For this review, use the dimensioned drawing (mm, ordinates from the lowest corner) and the shaded views. Coordinates: 2 decimals unless noted, no trailing zeros. Order: outer loops, then holes, each group sorted by start corner. A loop starts at its lowest first (then second) coordinate and runs counter-clockwise, first axis right, second up. Notation, with made-up numbers: M -15.75,-27 L 23.25,-27 A23 ccw 23.25,3 Z; hole C 32.5,-30.75 d10. An arc over 180 degrees is marked long. Use CSV: the item, a comma, the result in double quotes.
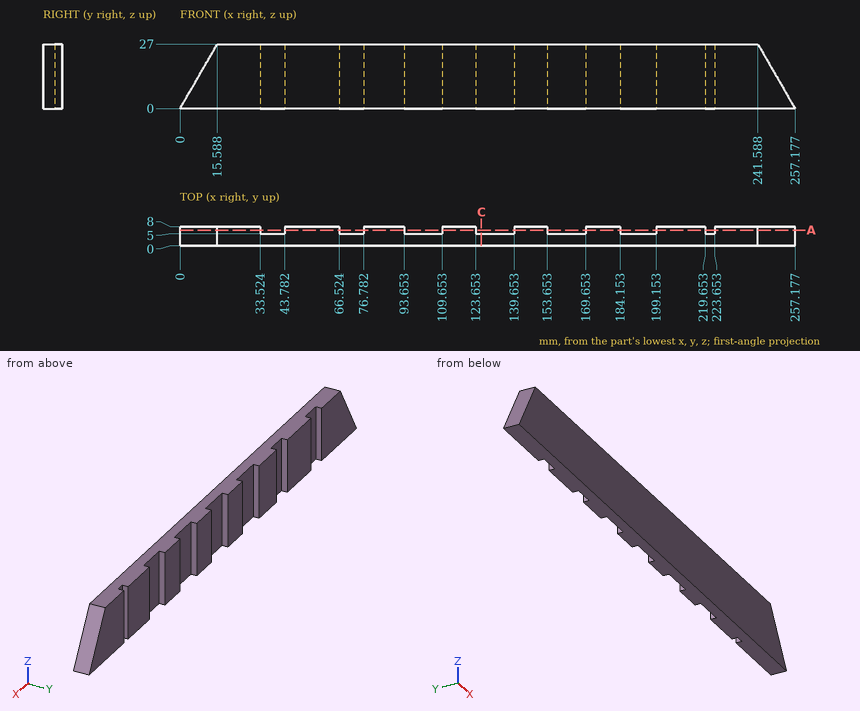
Item 1: Add section A-A on y = 6.5. State how many separate pieces and enclosed holes the cut face has, and give its area (3 significant figures).
Solutions:
separate pieces,"8"
enclosed holes,"0"
area,"4,160 mm^2"
Item 2: Clearance check with flat-ended pins moving along their axes: pin 1 Ø1.5 at (x, y) = (30.5, 6) entering from -Z; pin 2 Ø3.5 at (y, z) = (6.5, 7.5) entering from -X; pin 3 Ø0.9 at (y, z) = (6, 7.5) entering from -X; pin 4 Ø1.5 at (y, z) = (7, 13) entering from -X. State where each tip first meets the part, or that it passes through.
Solutions:
pin 1,"z = 0"
pin 2,"x = 3.32"
pin 3,"x = 4.07"
pin 4,"x = 7.07"
Item 3: Add section C-C on x = 126. State the section outline as (y, z) points.
Solutions:
outline,"M 0,0 L 5,0 L 5,27 L 0,27 Z"
Item 4: To check wall thickness, follow line 1 along Y through (x, z) = (95, 18.5); line 2 along X through (y, z) = (0.75, 22.25) (1 decimal); line 3 along X through (y, z) = (0.5, 14.5) (1 decimal). State the ranges of each line that lie inside material, in increasing order. Write a range as [from, to].
Solutions:
line 1,"[0, 5]"
line 2,"[12.8, 244.3]"
line 3,"[8.4, 248.8]"
